The listing builds one solid part. Answer for the finished solid, in the listing's coordinates (mm). A direction names the side the tool comes from. Round coordinates to 2 decimals unless told otherwise and drop trailing zeros. Write each loop counter-clockwise with the first axis right and the second up, starting at its lowest first coordinate (ties: lowest second). Pieces come first, ordered by that corner, then holes.
Item 1: Find section C-C on y = 56.5. Give the vertices of the cut face in (x, z), then the cut area to 3 significant figures.
Item 2: Find section D-D on y = 16. Give the vertices of the cut face in (x, z).
Item 3: Find the intervals of material crossed by probe 1 along X at (y, z) = (44, 0.55); probe 2 along X at (y, z) = (58.5, 1.3); probe 3 along X at (y, z) = (36, 0.85), in increasing order.
Item 4: A tool of negligible diameter and unlimited length cuts with its end or side. For faces 1 (the face through (7, 42.9, 0)), 2 (the face through (-1, -1, 0)), 3 (the face through (26.57, 63.02, 0.99)), 4 (the face through (37.5, 48, 0)), from which of +Z, -Z, +X, -X, +Y, -Y can it reach the whole face along a straight path? Write none if from no direction.
Item 5: Find section B-B on z = -0.7. Give the vertices of the cut face in (x, y).
Item 6: For a pull along Y with two mould halves and no side action, classify faces 5 (the face through (22.5, 39, 1)), 6 (the face through (22.5, 56, 0)), 7 (the face through (-0.361, 40.645, 0.028)) as +Y half, -Y half, draft (parallel to the pull), parting line (faces both ways), or undercut.
Item 7: Find section A-A on x = 8.5. Give the vertices of the cut face in (y, z), then the cut area to 3 significant figures.
Item 8: Each of these flat-tipped pins is pushed along its axis until it touches: pin 1 (2 mm diameter, centred on x = 48, z = -0.5, fed in from +Y); pin 2 (1 mm diameter, centred on x = 16.5, z = -1.5, fed in from -Y); pin 3 (1 mm diameter, centred on y = 30.5, z = 1, fed in from +X). Where does it stop, or does it pass through?
```python
from build123d import *

# Parameters (mm, degrees)
F1_DEPTH = 2
F3_DEPTH = 2
F5_DEPTH = 2
F7_DEPTH = 2
F9_DEPTH = 2


with BuildPart() as f1:
    # F0 (on Top) → F1 (new body)
    with BuildSketch(Plane.XY):
        with BuildLine():
            Line((-2.5, -2.5), (0, 0))
            Line((0, 0), (0, 25.4))
            Line((0, 25.4), (76.2, 25.4))
            Line((76.2, 25.4), (78.7, 27.9))
            Line((78.7, 27.9), (37.5, 27.9))
            Line((37.5, 27.9), (37.5, 67.17051))
            Line((37.5, 67.17051), (35, 67.17051))
            Line((35, 67.17051), (30, 67.17051))
            ThreePointArc((30, 67.17051), (24.696699, 64.973811), (22.5, 59.67051))
            Line((22.5, 59.67051), (22.5, 52.17051))
            Line((22.5, 52.17051), (17.5, 52.17051))
            ThreePointArc((17.5, 52.17051), (12.196699, 49.973811), (10, 44.67051))
            Line((10, 44.67051), (10, 42.9))
            Line((10, 42.9), (5, 42.9))
            ThreePointArc((5, 42.9), (-0.303301, 40.703301), (-2.5, 35.4))
            Line((-2.5, 35.4), (-2.5, 27.9))
            Line((-2.5, 27.9), (-2.5, -2.5))
        make_face()
        with BuildLine():
            Line((5.5, 40.4), (10, 40.4))
            Line((10, 40.4), (10, 27.9))
            Line((10, 27.9), (0, 27.9))
            Line((0, 27.9), (0, 34.9))
            ThreePointArc((0, 34.9), (1.610913, 38.789087), (5.5, 40.4))
        make_face(mode=Mode.SUBTRACT)
        with BuildLine():
            Line((18, 49.67051), (22.5, 49.67051))
            Line((22.5, 49.67051), (22.5, 27.9))
            Line((22.5, 27.9), (12.5, 27.9))
            Line((12.5, 27.9), (12.5, 44.17051))
            ThreePointArc((12.5, 44.17051), (14.110913, 48.059597), (18, 49.67051))
        make_face(mode=Mode.SUBTRACT)
        with BuildLine():
            Line((30.5, 64.67051), (35, 64.67051))
            Line((35, 64.67051), (35, 27.9))
            Line((35, 27.9), (25, 27.9))
            Line((25, 27.9), (25, 59.17051))
            ThreePointArc((25, 59.17051), (26.610913, 63.059597), (30.5, 64.67051))
        make_face(mode=Mode.SUBTRACT)
    extrude(amount=F1_DEPTH)

    # F2 (on face) → F3 (join)
    with BuildSketch(Plane(origin=(0, 0, 0), x_dir=(1, 0, 0), z_dir=(0, 0, -1))):
        with BuildLine():
            Line((0, 0), (-2.5, 2.5))
            Line((-2.5, 2.5), (-2.5, -35.4))
            ThreePointArc((-2.5, -35.4), (-0.303301, -40.703301), (5, -42.9))
            Line((5, -42.9), (10, -42.9))
            Line((10, -42.9), (10, -44.67051))
            ThreePointArc((10, -44.67051), (12.196699, -49.973811), (17.5, -52.17051))
            Line((17.5, -52.17051), (22.5, -52.17051))
            Line((22.5, -52.17051), (22.5, -59.67051))
            ThreePointArc((22.5, -59.67051), (24.696699, -64.973811), (30, -67.17051))
            Line((30, -67.17051), (37.5, -67.17051))
            Line((37.5, -67.17051), (37.5, -27.9))
            Line((37.5, -27.9), (78.7, -27.9))
            Line((78.7, -27.9), (76.2, -25.4))
            Line((76.2, -25.4), (0, -25.4))
            Line((0, -25.4), (0, 0))
        make_face()
    extrude(amount=F3_DEPTH)

    # F4 (on face) → F5 (join)
    with BuildSketch(Plane.XY):
        with BuildLine():
            Line((3.75, 34.375425), (3.75, 27.9))
            Line((3.75, 27.9), (6.25, 27.9))
            Line((6.25, 27.9), (6.25, 34.375425))
            ThreePointArc((6.25, 34.375425), (5.883883, 35.259308), (5, 35.625425))
            ThreePointArc((5, 35.625425), (4.116117, 35.259308), (3.75, 34.375425))
        make_face()
    extrude(amount=F5_DEPTH)

    # F6 (on face) → F7 (join)
    with BuildSketch(Plane.XY):
        with BuildLine():
            Line((16.25, 41.65), (16.25, 27.9))
            Line((16.25, 27.9), (18.75, 27.9))
            Line((18.75, 27.9), (18.75, 41.65))
            ThreePointArc((18.75, 41.65), (18.383883, 42.533883), (17.5, 42.9))
            ThreePointArc((17.5, 42.9), (16.616117, 42.533883), (16.25, 41.65))
        make_face()
    extrude(amount=F7_DEPTH)

    # F8 (on face) → F9 (join)
    with BuildSketch(Plane.XY):
        with BuildLine():
            Line((28.75, 50.92051), (28.75, 27.9))
            Line((28.75, 27.9), (31.25, 27.9))
            Line((31.25, 27.9), (31.25, 50.92051))
            ThreePointArc((31.25, 50.92051), (30.883883, 51.804393), (30, 52.17051))
            ThreePointArc((30, 52.17051), (29.116117, 51.804393), (28.75, 50.92051))
        make_face()
    extrude(amount=F9_DEPTH)


solid = f1.part
```
Check values:
1. outline: (22.5, -2) - (37.5, -2) - (37.5, 2) - (35, 2) - (35, 0) - (25, 0) - (25, 2) - (22.5, 2) - close
1. area: 40.0 mm2
2. outline: (-2.5, -2) - (0, -2) - (0, 2) - (-2.5, 2) - close
3. probe 1: x = 10 to 12.5, 22.5 to 25, 28.75 to 31.25, 35 to 37.5
3. probe 2: x = 22.5 to 25, 35 to 37.5
3. probe 3: x = -2.48 to 0.11, 10 to 12.5, 16.25 to 18.75, 22.5 to 25, 28.75 to 31.25, 35 to 37.5
4. face 1: +Z, -Z, -X, +Y
4. face 2: +Z, -Z, +X, -Y
4. face 3: +Z
4. face 4: +Z, -Z, +X, +Y
5. outline: (-2.5, -2.5) - (0, 0) - (0, 25.4) - (76.2, 25.4) - (78.7, 27.9) - (37.5, 27.9) - (37.5, 67.17) - (30, 67.17) arc R7.5 ccw to (22.5, 59.67) - (22.5, 52.17) - (17.5, 52.17) arc R7.5 ccw to (10, 44.67) - (10, 42.9) - (5, 42.9) arc R7.5 ccw to (-2.5, 35.4) - close
6. face 5: undercut
6. face 6: draft
6. face 7: +Y half
7. outline: (25.4, -2) - (42.9, -2) - (42.9, 2) - (40.4, 2) - (40.4, 0) - (27.9, 0) - (27.9, 2) - (25.4, 2) - close
7. area: 45.0 mm2
8. pin 1: stops at y = 27.9
8. pin 2: stops at y = 25.4
8. pin 3: stops at x = 37.5
